```python
from build123d import *

# Parameters (mm, degrees)
F0_W = 6
F0_H = 45
F2_W = 16.5
F2_H = 12
F4_R = 2


with BuildPart() as f1:
    # F0 (on Front) → F1 (revolve)
    with BuildSketch(Plane.XZ):
        with Locations((32, 0)):
            Rectangle(F0_W, F0_H)
    revolve(axis=Axis((0, 0, 12.074299), (0, 0, -1)))

    # F2 (on Front) → F3 (revolve)
    with BuildSketch(Plane.XZ):
        with Locations((20.75, 0)):
            Rectangle(F2_W, F2_H)
    revolve(axis=Axis((0, 0, 3.15167), (0, 0, -1)))

    # F4
    f4_edges = [f1.edges().sort_by_distance(p)[0] for p in [
        (-29, 0, 6),
        (-29, 0, -6),
    ]]
    fillet(f4_edges, radius=F4_R)


solid = f1.part
```
Work out the finished part from the listing and answer in its coordinate system (mm). A direction names the side the tool comes from. Round coordinates to 2 decimals unless told otherwise and drop trailing zeros. Write each loop counter-clockwise with the first axis right and the second up, starting at its lowest first coordinate (ties: lowest second). Pieces come first, ordered by that corner, then holes. Notation, with made-up numbers: (8.25, 45) - (24.25, 45) arc R18 ccw to (24.25, 50) - close; hole circle Ø5 at (68, -9). An arc over 180 degrees is marked (long way). Return JSON: item names as keys, results as strings. Group by question number.
Q1. The mould has two halves that part along Y. Classify faces 1 (the flat face through (13.1, -26.1, 22.5)), 2 (the cylindrical face through (-28, 21, 0)), 3 (the flat face through (-12, 6, 6)): released by +Y, released by -Y, zero draft, split by the parting line, or undercut.
Q2. For faces 4 (the flat face through (-12, 6, -6)), 5 (the cylindrical face through (13.38, 25.73, 15.35)), 6 (the cylindrical face through (11.923, -3.755, 0.084)), determine the directions among +Z, -Z, +X, -X, +Y, -Y from which every point of the face is accessible in a straight line to the end or side of a thin tool.
Q3. The part is cut by section A-A on x = 0. Write down the section's boundary in (y, z).
Q4. The part is cut by section D-D on z = -4.5. Write down the section's boundary in (x, y), then the cut area to 3 significant figures.
Q5. Each of these flat-tipped pins is pushed along its axis until it touches: pin 1 Ø1 at (y, z) = (-5, -4.5) entering from -X; pin 2 Ø10 at (y, z) = (-27.5, -14) entering from -X; pin 3 Ø2 at (x, z) = (12.5, -1.5) entering from -Y; pin 4 Ø12 at (x, y) = (-24, 2.5) entering from -Z. Where does it stop, or does it pass through?
Q6. The part is cut by section C-C on z = -12.5. Write down the section's boundary in (x, y), then the cut area to 3 significant figures.
Q7. Find the intervals of material crossed by L1, parallel to Y at x = 0, z = 19.5; L2, parallel to X at y = 0, z = 3, in increasing order.
Solved:
{
 "1": {"face 1": "zero draft", "face 2": "split by the parting line", "face 3": "undercut"},
 "2": {"face 4": "-Z", "face 5": "+Z", "face 6": "+Z, -Z"},
 "3": {"outline": "(-35, -22.5) - (-29, -22.5) - (-29, -8) arc R2 cw to (-27, -6) - (-12.5, -6) - (-12.5, 6) - (-27, 6) arc R2 cw to (-29, 8) - (-29, 22.5) - (-35, 22.5) - close; (12.5, -6) - (27, -6) arc R2 cw to (29, -8) - (29, -22.5) - (35, -22.5) - (35, 22.5) - (29, 22.5) - (29, 8) arc R2 cw to (27, 6) - (12.5, 6) - close"},
 "4": {"outline": "circle Ø70 at (0, 0); hole circle Ø25 at (0, 0)", "area": "3,360 mm²"},
 "5": {"pin 1": "x = -34.71", "pin 2": "x = -26.81", "pin 3": "y = -33.06", "pin 4": "z = -22.5"},
 "6": {"outline": "circle Ø70 at (0, 0); hole circle Ø58 at (0, 0)", "area": "1,210 mm²"},
 "7": {"L1": "-35 to -29, 29 to 35", "L2": "-35 to -12.5, 12.5 to 35"}
}
